Read the model definition and answer for the solid it produces. Units are mm, in the model's axes. A direction names the side the tool comes from. Coordinates: 2 decimals unless noted, no trailing zeros. Order: outer loops, then holes, each group sorted by start corner. A loop starts at its lowest first (then second) coordinate and runs counter-clockwise, first axis right, second up.
```python
from build123d import *

# Parameters (mm, degrees)
F0_R     = 25
F1_DEPTH = 20
F2_START = 20
F2_DEPTH = 60


with BuildPart() as f1:
    # F0 (on Front) → F1 (new body)
    with BuildSketch(Plane.XZ):
        with BuildLine():
            Line((-39.0416272934, 230.1646211462), (-127.893426815, 148.9686369788))
            ThreePointArc((-127.893426815, 148.9686369788), (1.8429896211, -196.3287722547), (125.0743198764, 151.3433114916))
            Line((125.0743198764, 151.3433114916), (39.0416272934, 230.1646211462))
            ThreePointArc((39.0416272934, 230.1646211462), (0, 253.7630542683), (-39.0416272934, 230.1646211462))
        make_face()
        with BuildLine():
            ThreePointArc((118.5096726545, 143.7953144771), (1.7986083479, -186.3287417074), (-121.2634079203, 141.480814522))
            Line((-121.2634079203, 141.480814522), (-30.9161716853, 224.0433827807))
            ThreePointArc((-30.9161716853, 224.0433827807), (-0.0030944403, 243.7630541279), (30.9135618095, 224.0489944464))
            Line((30.9135618095, 224.0489944464), (118.5096726545, 143.7953144771))
        make_face(mode=Mode.SUBTRACT)
        with BuildLine():
            Line((-30.9161716853, 224.0433827807), (-121.2634079203, 141.480814522))
            ThreePointArc((-121.2634079203, 141.480814522), (1.7986083479, -186.3287417074), (118.5096726545, 143.7953144771))
            Line((118.5096726545, 143.7953144771), (30.9135618095, 224.0489944464))
            ThreePointArc((30.9135618095, 224.0489944464), (-0.0030944403, 243.7630541279), (-30.9161716853, 224.0433827807))
        make_face()
        Circle(F0_R, mode=Mode.SUBTRACT)
    extrude(amount=F1_DEPTH)

    # F0 (on Front) → F2 (join)
    with BuildSketch(Plane.XZ.offset(F2_START)):
        with BuildLine():
            Line((-39.0416272934, 230.1646211462), (-127.893426815, 148.9686369788))
            ThreePointArc((-127.893426815, 148.9686369788), (1.8429896211, -196.3287722547), (125.0743198764, 151.3433114916))
            Line((125.0743198764, 151.3433114916), (39.0416272934, 230.1646211462))
            ThreePointArc((39.0416272934, 230.1646211462), (0, 253.7630542683), (-39.0416272934, 230.1646211462))
        make_face()
        with BuildLine():
            ThreePointArc((118.5096726545, 143.7953144771), (1.7986083479, -186.3287417074), (-121.2634079203, 141.480814522))
            Line((-121.2634079203, 141.480814522), (-30.9161716853, 224.0433827807))
            ThreePointArc((-30.9161716853, 224.0433827807), (-0.0030944403, 243.7630541279), (30.9135618095, 224.0489944464))
            Line((30.9135618095, 224.0489944464), (118.5096726545, 143.7953144771))
        make_face(mode=Mode.SUBTRACT)
    extrude(amount=F2_DEPTH)


solid = f1.part
```
1) A cutting plane is placed at C-C, the plane y = -38. Determine the outline of the cut face in (x, z).
A:
outline: (-127.89, 148.97) arc R196.34 ccw (long way) to (125.07, 151.34) - (39.04, 230.16) arc R44.09 ccw to (-39.04, 230.16) - close; hole (-121.26, 141.48) arc R186.34 ccw (long way) to (118.51, 143.8) - (30.91, 224.05) arc R34.09 ccw to (-30.92, 224.04) - close
2) Straight lines are drawn through the part: line 1 (Z direction, x = 0, y = -7.25); line 2 (X direction, y = -56, z = 0); line 3 (Z direction, x = -1, y = -15). For each, find the intervals that lie inside material, in ascending order.
A:
line 1: z = -196.34 to -25, 25 to 253.76
line 2: x = -196.34 to -186.34, 186.34 to 196.34
line 3: z = -196.33 to -24.98, 24.98 to 253.75
3) A cutting plane is placed at B-B, the plane x = 0. Determine the outline of the cut face in (y, z), and give its area (3 significant figures).
A:
outline: (-80, -196.34) - (0, -196.34) - (0, -25) - (-20, -25) - (-20, -186.34) - (-80, -186.34) - close; (-80, 243.76) - (-20, 243.76) - (-20, 25) - (0, 25) - (0, 253.76) - (-80, 253.76) - close
area: 9,200 mm2
4) A cutting plane is placed at D-D, the plane x = -171. Determine the outline of the cut face in (y, z), and give its area (3 significant figures).
A:
outline: (-80, -96.47) - (0, -96.47) - (0, 96.47) - (-80, 96.47) - (-80, 74.03) - (-20, 74.03) - (-20, -74.03) - (-80, -74.03) - close
area: 6,550 mm2
5) A cutting plane is placed at A-A, the plane z = 0. Determine the outline of the cut face in (x, y).
A:
outline: (-196.34, -80) - (-186.34, -80) - (-186.34, -20) - (-25, -20) - (-25, 0) - (-196.34, 0) - close; (25, -20) - (186.34, -20) - (186.34, -80) - (196.34, -80) - (196.34, 0) - (25, 0) - close
6) Flat-ended cylindrical pins translate along their axes: pin 1 Ø8 at (x, y) = (-40, -18) entering from -Z; pin 2 Ø4 at (x, z) = (129, -117.5) entering from -Y; pin 3 Ø10 at (y, z) = (-64, 41.5) entering from +X. Find the tip coordinate at first contact, or state that the pin passes through.
A:
pin 1: stops at z = -193.01
pin 2: stops at y = -20
pin 3: stops at x = 192.91
7) Which of the six approach directions +Z, -Z, +X, -X, +Y, -Y give full straight-line access (tool end or side, diameter ignored) to faces 1 (the cylindrical face through (-4.868, -39.44, -196.277)), 2 (the cylindrical face through (8.17, -49.58, -186.16))?
A:
face 1: +Y, -Y
face 2: -Y
8) Determine the mould class of faces 3 (the flat face through (-82.846, -39.44, 190.135)), 4 (the flat face through (74.1, -49.58, 184.48)), 5 (the flat face through (-117, -80, 146)) for opening direction Z: pulls with the +Z half, pulls with the -Z half, needs draft (parallel to the pull), parting line crosses it, or undercut.
A:
face 3: pulls with the +Z half
face 4: undercut
face 5: needs draft
